CAD build for the part. Positions are in the model's coordinates, mm. A direction names the side the tool comes from. Coordinates: 2 decimals unless noted, no trailing zeros. Loops run counter-clockwise (first coordinate to the right, second up) from the corner with the lowest first, then second, coordinate; pieces in that order, holes last. Notation, with made-up numbers: (84.25, 24.25) -> (107.25, 24.25) arc R33 cw to (107.25, 61.25) -> close; hole circle Ø10 at (71.25, -32.75). An arc over 180 degrees is marked (long way). Write each question's results on one line, items separated by ' | '.
```python
from build123d import *
from build123d.topology import SkipClean

# Parameters (mm, degrees)
SKETCH1_R               = 45
BOSS_EXTRUDE1_DEPTH     = 35
CUT_EXTRUDE1_DEPTH      = 30
BOSS_EXTRUDE2_START     = 20
SKETCH3_R               = 50
SKETCH3_R_2             = 45
BOSS_EXTRUDE2_DEPTH     = 20
SKETCH4_R               = 22.5
BOSS_EXTRUDE3_DEPTH     = 108
SKETCH5_R               = 62.5
BOSS_EXTRUDE4_DEPTH     = 3
CUT_EXTRUDE2_DEPTH      = 283.934340716
CUT_EXTRUDE2_DEPTH_BACK = 283.934340716
SKETCH6_R               = 16.5
CHAMFER1_START          = -20
CHAMFER1_DEPTH          = 20
BOSS_EXTRUDE5_START     = 20
BOSS_EXTRUDE5_DEPTH     = 20
CHAMFER3_START          = -59.701385296
CHAMFER3_DEPTH          = 31.623598411
CHAMFER3_START_2        = -32.908910756
CHAMFER3_2_DEPTH        = 24.320342802
CHAMFER3_START_3        = -75.100600507
CHAMFER3_3_DEPTH        = 17.710815412
CHAMFER3_START_4        = -108
CHAMFER3_4_DEPTH        = 20.0000001
CUT_EXTRUDE3_START      = 20
CUT_EXTRUDE3_DEPTH      = 20
CUT_EXTRUDE4_DEPTH      = 3
FILLET2_R               = 5


with BuildPart() as part:
    # Sketch1 → Boss-Extrude1 (new body)
    with BuildSketch(Plane(origin=(0, 0, 0), x_dir=(1, 0, 0), z_dir=(0, 1, 0))):
        Polygon((46.859255168, 63.80155033), (-83.545615043, 63.80155033), (-97.357476794, 66.23695421), (-86.281022646, 129.054647247), (-78.894964498, 127.752285914), (-74.254340533, 154.070572239), (0, 208.019508525), (75.819867549, 152.933150283), align=None)
        with Locations(Location((0, 127.60310066, 0), (0, 0, 90))):
            Circle(SKETCH1_R, mode=Mode.SUBTRACT)
    extrude(amount=BOSS_EXTRUDE1_DEPTH)

    # Sketch2 → Cut-Extrude1 (cut)
    with BuildSketch(Plane(origin=(0, 35, 0), x_dir=(1, 0, 0), z_dir=(0, 1, 0))):
        Polygon((69.942015026, 151.023320226), (0, 201.839168637), (-69.681093857, 151.212890552), (-74.839166621, 121.960006261), (-82.225224769, 123.262367593), (-91.56519714, 70.292752087), (-83.108171726, 68.80155033), (43.226542528, 68.80155033), align=None)
    extrude(amount=-CUT_EXTRUDE1_DEPTH, mode=Mode.SUBTRACT)

    # Sketch3 → Boss-Extrude2 (add)
    with BuildSketch(Plane.XZ.offset(BOSS_EXTRUDE2_START)):
        with Locations(Location((0, -127.60310066, 0), (0, 0, 270))):
            Circle(SKETCH3_R)
        with Locations(Location((0, -127.60310066, 0), (0, 0, 270))):
            Circle(SKETCH3_R_2, mode=Mode.SUBTRACT)
    extrude(amount=-BOSS_EXTRUDE2_DEPTH)

    # Sketch4 → Boss-Extrude3 (add)
    with BuildSketch(Plane.XZ):
        with Locations(Location((-61.853227661, -94.828442341, 0), (0, 0, 354.769849307))):
            Circle(SKETCH4_R)
    extrude(amount=BOSS_EXTRUDE3_DEPTH)

    # Sketch5 → Boss-Extrude4 (add)
    with BuildSketch(Plane.XZ.offset(108)):
        with Locations(Location((-61.853227661, -94.828442341, 0), (0, 0, 270))):
            Circle(SKETCH5_R)
    extrude(amount=BOSS_EXTRUDE4_DEPTH)

    # Sketch6 → Cut-Extrude2 (cut, two sides: drawn at the far end of the back side and taken through both)
    with BuildSketch(Plane.XZ.offset(111).offset(-CUT_EXTRUDE2_DEPTH_BACK)):
        with Locations(Location((-61.853227661, -94.828442341, 0), (0, 0, 270))):
            Circle(SKETCH6_R)
    extrude(amount=CUT_EXTRUDE2_DEPTH + CUT_EXTRUDE2_DEPTH_BACK, mode=Mode.SUBTRACT)

    # Chamfer1: read off the stored shape, not the designer's step
    # Chamfer1 outline → Chamfer1 (add)
    with BuildSketch(Plane(origin=(0, 0, 0), x_dir=(1, 0, 0), z_dir=(0, 1, 0)).offset(CHAMFER1_START)):
        with BuildLine():
            ThreePointArc((-47.573643712, 112.216469321), (-49.998001272, 128.050167568), (-47.290893773, 143.837981816))
            Line((-47.290893773, 143.837981816), (-60.85462884, 117.306271426))
            ThreePointArc((-60.85462884, 117.306271426), (-53.801380758, 115.838386688), (-47.573643712, 112.216469321))
        make_face()
        with BuildLine():
            Line((-42.693487755, 83.032071427), (-13.123343442, 79.356050419))
            ThreePointArc((-13.123343442, 79.356050419), (-27.706953652, 85.981895496), (-39.446904898, 96.879466533))
            ThreePointArc((-39.446904898, 96.879466533), (-39.947247216, 89.692488608), (-42.693487755, 83.032071427))
        make_face()
    extrude(amount=CHAMFER1_DEPTH)

    # Sketch7 → Boss-Extrude5 (add)
    with SkipClean():  # the faces are left unmerged after this step: merging them gives an invalid solid
        with BuildSketch(Plane(origin=(0, -108, 0), x_dir=(1, 0, 0), z_dir=(0, 1, 0)).offset(BOSS_EXTRUDE5_START)):
            with BuildLine():
                Line((-70.209230864, 52.9494319), (-20.454240978, 48.005649797))
                ThreePointArc((-20.454240978, 48.005649797), (-22.061100088, 46.632627344), (-23.713465467, 45.314721618))
                Line((-23.713465467, 45.314721618), (-70.50585779, 49.964132507))
                Line((-70.50585779, 49.964132507), (-70.209230864, 52.9494319))
            make_face()
            with BuildLine():
                Line((-64.077929608, 72.438696893), (-6.054139097, 66.673305768))
                ThreePointArc((-6.054139097, 66.673305768), (-5.354795719, 68.104348565), (-4.69214598, 69.552747672))
                Line((-4.69214598, 69.552747672), (-52.611335155, 74.314119956))
                ThreePointArc((-52.611335155, 74.314119956), (-58.221486515, 72.623477665), (-64.077929608, 72.438696893))
            make_face()
        extrude(amount=-BOSS_EXTRUDE5_DEPTH)

    # Chamfer3: read off the stored shape, not the designer's step
    # Chamfer3 outline → Chamfer3 (add)
    with SkipClean():  # the faces are left unmerged after this step: merging them gives an invalid solid
        with BuildSketch(Plane(origin=(0, 0, 0), x_dir=(0, 1, 0), z_dir=(0.9950997977115372, 0, 0.09887564206849853)).offset(CHAMFER3_START)):
            Polygon((-108, -68.747986192), (-108, -83.747986192), (-93, -68.747986192), align=None)
            Polygon((-108, -27.747986192), (-108, -42.747986192), (-93, -42.747986192), align=None)
        extrude(amount=CHAMFER3_DEPTH)

    # Chamfer3 2 outline → Chamfer3 2 (add)
    with SkipClean():  # the faces are left unmerged after this step: merging them gives an invalid solid
        with BuildSketch(Plane(origin=(0, 0, 0), x_dir=(0, 1, 0), z_dir=(0.9950997977115372, 0, 0.09887564206849853)).offset(CHAMFER3_START_2)):
            Polygon((-108, -68.747986192), (-108, -83.747986192), (-93, -68.747986192), align=None)
        extrude(amount=CHAMFER3_2_DEPTH)

    # Chamfer3 3 outline → Chamfer3 3 (add)
    with SkipClean():  # the faces are left unmerged after this step: merging them gives an invalid solid
        with BuildSketch(Plane(origin=(0, 0, 0), x_dir=(0, 1, 0), z_dir=(0.9950997977115372, 0, 0.09887564206849853)).offset(CHAMFER3_START_3)):
            Polygon((-108, -27.747986192), (-108, -42.747986192), (-93, -42.747986192), align=None)
        extrude(amount=CHAMFER3_3_DEPTH)

    # Chamfer3 4 outline → Chamfer3 4 (cut)
    with SkipClean():  # the faces are left unmerged after this step: merging them gives an invalid solid
        with BuildSketch(Plane(origin=(0, 0, 0), x_dir=(1, 0, 0), z_dir=(0, 1, 0)).offset(CHAMFER3_START_4)):
            with BuildLine():
                Line((-51.128200524, 89.240616922), (-51.879001502, 81.68443943))
                ThreePointArc((-51.879001502, 81.68443943), (-48.702503608, 84.863079484), (-46.501448484, 88.780891094))
                Line((-46.501448484, 88.780891094), (-51.128200524, 89.240616922))
            make_face()
            with BuildLine():
                ThreePointArc((-0.265846327, 84.186804289), (-2.029835327, 76.733920253), (-4.69214598, 69.552747672))
                Line((-4.69214598, 69.552747672), (-1.748980958, 69.260307324))
                Line((-1.748980958, 69.260307324), (-0.265846327, 84.186804289))
            make_face()
            with BuildLine():
                ThreePointArc((-23.713465467, 45.314721618), (-37.1988252, 37.396652892), (-52.227673534, 33.074100731))
                Line((-52.227673534, 33.074100731), (-25.196600099, 30.388224653))
                Line((-25.196600099, 30.388224653), (-23.713465467, 45.314721618))
            make_face()
        extrude(amount=CHAMFER3_4_DEPTH, mode=Mode.SUBTRACT)

    # Sketch9 → Cut-Extrude3 (cut)
    with SkipClean():  # the faces are left unmerged after this step: merging them gives an invalid solid
        with BuildSketch(Plane(origin=(0, -108, 0), x_dir=(1, 0, 0), z_dir=(0, 1, 0)).offset(CUT_EXTRUDE3_START)):
            Polygon((-61.020192816, 33.947747767), (-75.946689782, 35.430882398), (-74.463555151, 50.357379364), (-59.537058185, 48.874244733), align=None)
            Polygon((-56.551758792, 48.577617807), (-58.034893423, 33.651120841), (-38.132897469, 31.673608), (-36.649762838, 46.600104965), align=None)
            Polygon((-33.664463445, 46.303478039), (-35.147598076, 31.376981073), (-15.245602121, 29.399468232), (-13.76246749, 44.325965198), align=None)
            Polygon((-33.104139652, 87.449700478), (-34.587274283, 72.523203512), (-14.685278328, 70.54569067), (-13.202143697, 85.472187636), align=None)
            with BuildLine():
                Line((-36.089439045, 87.746327404), (-37.572573676, 72.819830438))
                Line((-37.572573676, 72.819830438), (-52.611335155, 74.314119956))
                ThreePointArc((-52.611335155, 74.314119956), (-44.996440318, 79.925465442), (-40.360787322, 88.170739412))
                Line((-40.360787322, 88.170739412), (-36.089439045, 87.746327404))
            make_face()
            with BuildLine():
                Line((-0.265846327, 84.186804289), (-10.216844304, 85.17556071))
                Line((-10.216844304, 85.17556071), (-11.699978935, 70.249063744))
                Line((-11.699978935, 70.249063744), (-4.69214598, 69.552747672))
                ThreePointArc((-4.69214598, 69.552747672), (-2.029835327, 76.733920253), (-0.265846327, 84.186804289))
            make_face()
        extrude(amount=-CUT_EXTRUDE3_DEPTH, mode=Mode.SUBTRACT)

    # Sketch10 → Cut-Extrude4 (cut)
    with SkipClean():  # the faces are left unmerged after this step: merging them gives an invalid solid
        with BuildSketch(Plane(origin=(-37.891198026, 0, -3.764965627), x_dir=(-0.09887564206850087, 0, 0.995099797711537), z_dir=(-0.995099797711537, 0, -0.09887564206850087))):
            Polygon((-42.747986192, -93), (-35.076363954, -108), (-30.076363954, -108), (-30.076363954, -93), align=None)
        extrude(amount=CUT_EXTRUDE4_DEPTH, mode=Mode.SUBTRACT)

    # Fillet2
    # the kernel refuses this fillet: 5 mm, written as the material it adds along each edge
    with BuildSketch(Plane(origin=(-70.50585779, -108, -49.964132507), x_dir=(-0.9950997977115372, 0, -0.09887564206849696), z_dir=(0.09887564206849697, 0, -0.9950997977115373))) as fillet2_piece_1:
        with BuildLine():
            CenterArc((FILLET2_R, FILLET2_R), FILLET2_R, 180, 90)
            Line((0, FILLET2_R), (0, 0))
            Line((0, 0), (FILLET2_R, 0))
        make_face()
    extrude(amount=3)


solid = part.part
```
Q1. Pull direction Y, two halves, no side cores. Call faces 5 (the flat face through (-86.83, 20.21, -97.15)), 6 (the flat face through (-48, 5, -121)), 7 (the flat face through (-30, -88, -71)): +Y half, -Y half, draft (parallel to the pull), parting line (faces both ways), or undercut.
Results are:
face 5: draft | face 6: +Y half | face 7: undercut
Q2. Which spindle directions (+Z, -Z, +X, -X, +Y, -Y) get a long thin tool onto all of the face, cutting with end or side? Do faces 1 (the flat face through (2, 0, -77)), 2 (the flat face through (35.461, 20.21, -176.076)), 3 (the flat face through (-90.35, 17.26, -65)), 4 (the flat face through (-28.12, -10.14, -81.22)). Say none if no direction does.
Results are:
face 1: none | face 2: +Y | face 3: +Z, -X, +Y | face 4: +Z
Q3. Cut at B-B on z = -186. Write the cut outline in (x, y), and give its area (3 significant figures).
Results are:
outline: (-30.31, 0) -> (30.31, 0) -> (30.31, 35) -> (21.8, 35) -> (21.8, 5) -> (-21.8, 5) -> (-21.8, 35) -> (-30.31, 35) -> close | area: 813 mm^2
Q4. Cut at C-C on x = 55. Write the cut outline in (y, z).
Results are:
outline: (0, -168.06) -> (35, -168.06) -> (35, -161.88) -> (5, -161.88) -> (5, -105.04) -> (35, -105.04) -> (35, -88.86) -> (0, -88.86) -> close
Q5. Drop flat-ended pins along their axis: pin 1 (1 mm diameter, centred on x = -68, y = -91.5, fed in from -Z); pin 2 (8.5 mm diameter, centred on x = -39.5, z = -48.5, fed in from +Y); pin 3 (15 mm diameter, centred on x = -38, y = 24, fed in from -Z). Give the stop position or say it passes through.
Results are:
pin 1: z = -116.61 | pin 2: y = -88 | pin 3: z = -185.86
Q6. Cut at A-A on x = 16. Write the cut outline in (y, z), and give its area (3 significant figures).
Results are:
outline: (-20, -174.97) -> (0, -174.97) -> (0, -196.39) -> (35, -196.39) -> (35, -190.21) -> (5, -190.21) -> (5, -169.66) -> (-20, -169.66) -> close; (-20, -85.54) -> (5, -85.54) -> (5, -68.8) -> (35, -68.8) -> (35, -63.8) -> (0, -63.8) -> (0, -80.23) -> (-20, -80.23) -> close | area: 790 mm^2
Q7. Wall check: L1, parallel to X at y = -81, z = -95.5; L2, parallel to Y at x = -79.5, z = -126.5; L3, parallel to X at y = 13, z = -147. Give the ranges that are in metal, low to high. Write a range as from..to.
Results are:
L1: -84.34..-78.34, -45.37..-39.36 | L2: -111..-108, 0..35 | L3: -75.5..-70.42, 68.63..73.89
Q8. Cut at D-D on y = -62. Write the cut outline in (x, z).
Results are:
outline: circle Ø45 at (-61.85, -94.83); hole circle Ø33 at (-61.85, -94.83)
